Input: part model. Units: mm. Frame: model coordinates. A direction names the side the tool comes from. Give positions to 0.01 mm unless a question says otherwise; leave off trailing zeros. Order: outer loops, then holes, each group sorted by start corner. A loop starts at its lowest first (then second) coordinate and runs counter-clockwise, first axis right, second up. Notation, with made-up numbers: (-22.75, 89.25) - (1.25, 89.25) arc R18 cw to (1.25, 111.25) - close; hole circle Ø8 at (-13.75, -12). An arc over 180 degrees is marked (long way). Use a Markdown table: item, result.
from build123d import *

# Parameters (mm, degrees)
SKETCH_1_R          = 1.25
SKETCH_1_R_2        = 1
SKETCH_1_R_3        = 2
EXTRUDE_1_DEPTH     = 2.5
EXTRUDE_2_DEPTH     = 10
EXTRUDE_START       = 2.5
EXTRUDE_4_DEPTH     = 2
FILLET_1_R          = 1
FILLET_2_R          = 6
EXTRUDE_START_2     = 7.5
SKETCH_2_W          = 2
SKETCH_2_H          = 16
EXTRUDE_5_DEPTH     = 7.5
SKETCH_3_W          = 7.5
SKETCH_3_H          = 5
EXTRUDE_6_DEPTH     = 14
SKETCH_4_R          = 1.6
CUT_EXTRUDE_1_DEPTH = 10
CUT_EXTRUDE_2_DEPTH = 10
CUT_EXTRUDE_3_DEPTH = 10
SKETCH_7_W          = 16
SKETCH_7_H          = 2.5
EXTRUDE_7_DEPTH     = 16
SKETCH_8_W          = 16
SKETCH_8_H          = 10.551633207
CUT_EXTRUDE_4_DEPTH = 7.5
CUT_EXTRUDE_5_DEPTH = 10
FILLET_3_R          = 2


with BuildPart() as part:
    # 草图1 → 凸台-拉伸1 (new body)
    with BuildSketch(Plane.XY):
        with BuildLine():
            Line((22, 6), (0, 6))
            ThreePointArc((0, 6), (-6, 0), (0, -6))
            Line((0, -6), (50, -6))
            Line((50, -6), (50, 13.5))
            ThreePointArc((50, 13.5), (48.681980515, 16.681980515), (45.5, 18))
            Line((45.5, 18), (26.5, 18))
            ThreePointArc((26.5, 18), (23.318019485, 16.681980515), (22, 13.5))
            Line((22, 13.5), (22, 6))
        make_face()
        with Locations((45.5, 13.5)):
            Circle(SKETCH_1_R, mode=Mode.SUBTRACT)
        with Locations((26.5, 13.5)):
            Circle(SKETCH_1_R, mode=Mode.SUBTRACT)
        Circle(SKETCH_1_R_2, mode=Mode.SUBTRACT)
        with Locations((5, 0)):
            Circle(SKETCH_1_R_2, mode=Mode.SUBTRACT)
        with Locations((36, 0)):
            Circle(SKETCH_1_R_3, mode=Mode.SUBTRACT)
    extrude(amount=EXTRUDE_1_DEPTH)

    # 草图1<3> → 凸台-拉伸2 (add)
    with BuildSketch(Plane.XY):
        Polygon((28, 9), (28, 6), (28, -6), (44, -6), (44, 9), (42, 9), (42, -4), (30, -4), (30, 9), align=None)
    extrude(amount=EXTRUDE_2_DEPTH)

    # 草图1<5> → 凸台-拉伸4 (add)
    with BuildSketch(Plane.XY.offset(EXTRUDE_START)):
        with BuildLine():
            ThreePointArc((26.5, 18), (22, 13.5), (26.5, 9))
            Line((26.5, 9), (26.5, 12.25))
            ThreePointArc((26.5, 12.25), (25.25, 13.5), (26.5, 14.75))
            Line((26.5, 14.75), (26.5, 18))
        make_face()
        with BuildLine():
            Line((45.5, 12.25), (45.5, 9))
            ThreePointArc((45.5, 9), (50, 13.5), (45.5, 18))
            Line((45.5, 18), (45.5, 14.75))
            ThreePointArc((45.5, 14.75), (46.75, 13.5), (45.5, 12.25))
        make_face()
    extrude(amount=EXTRUDE_4_DEPTH)

    # 圆角1
    fillet_1_edges = [part.edges().sort_by_distance(p)[0] for p in [
        (42, 9, 6.25),
        (30, 9, 6.25),
    ]]
    fillet(fillet_1_edges, radius=FILLET_1_R)

    # 圆角2
    fillet_2_edges = [part.edges().sort_by_distance(p)[0] for p in [
        (50, -6, 1.25),
        (22, 6, 1.25),
    ]]
    fillet(fillet_2_edges, radius=FILLET_2_R)

    # 草图2 → 凸台-拉伸5 (add)
    with BuildSketch(Plane.XY.offset(2.5).offset(EXTRUDE_START_2)):
        with Locations((43, 26)):
            Rectangle(SKETCH_2_W, SKETCH_2_H)
        with BuildLine():
            Line((43, 9), (44, 9))
            Line((44, 9), (44, 18))
            Line((44, 18), (42, 18))
            Line((42, 18), (42, 8))
            ThreePointArc((42, 8), (42.292893219, 8.707106781), (43, 9))
        make_face()
        with BuildLine():
            Line((28, 18), (28, 9))
            Line((28, 9), (29, 9))
            ThreePointArc((29, 9), (29.707106781, 8.707106781), (30, 8))
            Line((30, 8), (30, 18))
            Line((30, 18), (28, 18))
        make_face()
        with Locations((29, 26)):
            Rectangle(SKETCH_2_W, SKETCH_2_H)
    extrude(amount=-EXTRUDE_5_DEPTH)

    # 草图3 → 凸台-拉伸6 (add)
    with BuildSketch(Plane.ZY.offset(-28)):
        with Locations((6.25, 31.5)):
            Rectangle(SKETCH_3_W, SKETCH_3_H)
    extrude(amount=-EXTRUDE_6_DEPTH)

    # 草图4 → 切除-拉伸1 (cut)
    with BuildSketch(Plane(origin=(0, 34, 0), x_dir=(1, 0, 0), z_dir=(0, 1, 0))):
        with Locations(Location((33, -6.25, 0), (0, 0, 270))):
            Circle(SKETCH_4_R)
        with Locations(Location((39, -6.25, 0), (0, 0, 270))):
            Circle(SKETCH_4_R)
    extrude(amount=-CUT_EXTRUDE_1_DEPTH, mode=Mode.SUBTRACT)

    # 草图5 → 切除-拉伸2 (cut)
    with BuildSketch(Plane(origin=(0, 0, 0), x_dir=(-1, 0, 0), z_dir=(0, 0, -1))):
        Polygon((-30.670698378, 12.335500495), (-40.317654114, 12.335500495), (-35.634644198, 3.950389209), align=None)
    extrude(amount=-CUT_EXTRUDE_2_DEPTH, mode=Mode.SUBTRACT)

    # 草图6 → 切除-拉伸3 (cut)
    with BuildSketch(Plane(origin=(0, 0, 0), x_dir=(-1, 0, 0), z_dir=(0, 0, -1))):
        Polygon((-21.861162721, 0.94929577), (-21.861162721, -3.850507305), (-12.896241274, -3.850507305), align=None)
    extrude(amount=-CUT_EXTRUDE_3_DEPTH, mode=Mode.SUBTRACT)

    # 草图7 → 凸台-拉伸7 (add)
    with BuildSketch(Plane(origin=(0, 18, 0), x_dir=(1, 0, 0), z_dir=(0, 1, 0))):
        with Locations((36, -1.25)):
            Rectangle(SKETCH_7_W, SKETCH_7_H)
    extrude(amount=EXTRUDE_7_DEPTH)

    # 草图8 → 切除-拉伸4 (cut)
    with BuildSketch(Plane.XY.offset(10)):
        with Locations((36, 12.770298386)):
            Rectangle(SKETCH_8_W, SKETCH_8_H)
    extrude(amount=-CUT_EXTRUDE_4_DEPTH, mode=Mode.SUBTRACT)

    # 草图9 → 切除-拉伸5 (cut)
    with BuildSketch(Plane.XY.offset(2.5)):
        Polygon((33.245819602, 20.82286057), (40.232309823, 20.82286057), (33.245819602, 27.737325118), align=None)
    extrude(amount=-CUT_EXTRUDE_5_DEPTH, mode=Mode.SUBTRACT)

    # 圆角3
    fillet_3_edges = [part.edges().sort_by_distance(p)[0] for p in [
        (44, 34, 5),
        (28, 34, 5),
        (28, 18.046114989, 6.25),
        (28, 7.494481782, 6.25),
        (44, 18.046114989, 6.25),
        (44, 7.494481782, 6.25),
        (28, -6, 6.25),
        (44, -6, 6.25),
    ]]
    fillet(fillet_3_edges, radius=FILLET_3_R - 0.0001)  # a hair under: the kernel refuses the full size


solid = part.part
1. Mould query, pull axis X, two halves, no side actions, for faces 4 (the face through (21.861, -1, 1)), 5 (the face through (50, 7, 1)), 6 (the face through (24, 14, 4.5)). Classes: pulls with the +X half, pulls with the -X half, needs draft (parallel to the pull), parting line crosses it, or undercut.
Response:
| item | result |
|---|---|
| face 4 | undercut |
| face 5 | pulls with the +X half |
| face 6 | needs draft |
2. Section query A-A (z = 3.75). State how many separate pieces and enclosed holes the cut face has, then the cut area to 3 significant figures.
Response:
| item | result |
|---|---|
| separate pieces | 4 |
| enclosed holes | 0 |
| area | 254 mm^2 |
3. Section query B-B (y = 30). Return loops of the section in (x, z).
Response:
| item | result |
|---|---|
| outline | (28, 0) - (44, 0) - (44, 10) - (28, 10) - close; hole circle Ø3.2 at (33, 6.25); hole circle Ø3.2 at (39, 6.25) |
4. Set-up query: faces 1 (the face through (28.57, 18.65, 6.2)), 2 (the face through (42, 2, 6)), 3 (the face through (45, 18, 1)). Return all of +Z, -Z, +X, -X, +Y, -Y with unobstructed straight access to the full face (end or side cutting, diameter ignored); none if empty.
Response:
| item | result |
|---|---|
| face 1 | +Z, -X |
| face 2 | +Z |
| face 3 | +Z, -Z, +X, +Y |
5. Pin query (flat end, axial travel): pin 1 (2 mm diameter, centred on y = 17, z = 3.5, fed in from -X); pin 2 (1.5 mm diameter, centred on x = 20.5, y = 13.5, fed in from -Z); pin 3 (4 mm diameter, centred on y = 6.5, z = 6, fed in from +X); pin 4 (1.2 mm diameter, centred on y = -1, z = 1, fed in from -X). Return the tip coordinate at first contact, or that it passes through.
Response:
| item | result |
|---|---|
| pin 1 | stops at x = 22.76 |
| pin 2 | passes through |
| pin 3 | stops at x = 44 |
| pin 4 | stops at x = -5.99 |
6. Material intervals for line 1 along X through (y, z) = (32.15, 6.25); line 2 along X through (y, z) = (21, 7.5); line 3 along X through (y, z) = (13.5, 3.5), sorted ascending.
Response:
| item | result |
|---|---|
| line 1 | x = 28.01 to 31.4, 34.6 to 37.4, 40.6 to 43.99 |
| line 2 | x = 28 to 30, 42 to 44 |
| line 3 | x = 22 to 25.25, 46.75 to 50 |
7. Section query D-D (x = 11). Return loops of the section in (y, z).
Response:
| item | result |
|---|---|
| outline | (-6, 0) - (6, 0) - (6, 2.5) - (-6, 2.5) - close |
